The model under review builds one solid part; all positions refer to its coordinate system, in mm. A direction names the side the tool comes from. Round coordinates to 2 decimals unless told otherwise and drop trailing zeros. Loops run counter-clockwise (first coordinate to the right, second up) from the corner with the lowest first, then second, coordinate; pieces in that order, holes last. Notation, with made-up numbers: (58.25, 45) - (97.25, 45) arc R18 ccw to (97.25, 77) - close; hole circle Ø3 at (79, 20). An arc over 180 degrees is marked (long way). Answer as CSV lines item,"result".
Autodesk Inventor part; units mm, degrees
ref_plane "YZ Plane" through (0, 0, 0) normal (1, 0, 0) x (0, 1, 0)
ref_plane "XZ Plane" through (0, 0, 0) normal (0, 1, 0) x (-1, 0, 0)
ref_plane "XY Plane" through (0, 0, 0) normal (0, 0, 1) x (1, 0, 0)
sketch "Sketch1" plane through (0, 0, 0) normal (1, 0, 0) x (0, 1, 0)
  line L0 (15, 25) -> (-5, 25)
  line L1 (-5, 25) -> (-5, -25)
  line L2 (-5, -25) -> (15, -25)
  line L3 (15, -25) -> (0, -10)
  line L4 (0, -10) -> (0, 10)
  line L5 (0, 10) -> (15, 25)
  line L6 (0, 0) -> (-5, 0) construction
  circle A0 centre (5, -20) radius 2
  circle A1 centre (5, 20) radius 2
  dimension "d0" = 50
  dimension "d1" = 45
  dimension "d2" = 5
  dimension "d4" = 40
  dimension "d5" = 4
  dimension "d6" = 20
  dimension "d7" = 5
  dimension "d8" = 15
extrude "Extrusion1" add sketch "Sketch1" along normal blind 5
sketch "Sketch2" plane through (0, 0, 0) normal (-1, 0, 0) x (0, 0, 1)
  line L0 (25, -5) -> (-25, -5)
  line L1 (-25, -5) -> (25, -5)
  line L2 (25, -5) -> (25, 0)
  line L3 (25, 0) -> (-25, 0)
  line L4 (-25, 0) -> (-25, -5)
  point P0 (0, 0)
extrude "Extrusion2" add sketch "Sketch2" along normal blind 10
mirror "Mirror1" about plane through (-10, -2.5, 0) normal (-1, 0, 0)
sketch "Sketch3" plane through (0, 0, 10) normal (0, 1, 0) x (1, 0, 0)
  line L0 (-20, 0) -> (-20, -15) construction
  line L1 (0, 20) -> (5, 20) construction
  line L2 (-20, 0) -> (0, 20) construction
  line L3 (-20, 35) -> (-20, 20) construction
  line L4 (0, 0) -> (5, 0) construction
  line L5 (-20, 20) -> (0, 0) construction
  circle A0 centre (-10, 10) radius 2
  point P0 (0, 10)
  dimension "d13" = 4
extrude "Extrusion3" cut sketch "Sketch3" against normal blind 2
sketch "Sketch4" plane through (0, 0, 10) normal (0, 1, 0) x (1, 0, 0)
  circle A0 centre (-10, 10) radius 2
  circle A1 centre (-10, 10) radius 1
  point P0 (0, 10)
  dimension "d16" = 2
extrude "Extrusion4" cut sketch "Sketch4" against normal through all contours A1
equation "\"d7\" = 0.333333 * d8"
properties part number "lower fan mount"
1. Clearance check with flat-ended pins moving along their axes: pin 1 (1 mm diameter, centred on x = -3, z = 19.5, fed in from +Y); pin 2 (12 mm diameter, centred on y = 9, z = -17.5, fed in from -X); pin 3 (2 mm diameter, centred on x = -10, z = -0.5, fed in from +Y); pin 4 (3 mm diameter, centred on y = 2.5, z = 2.5, fed in from +X). State where each tip first meets the part, or that it passes through.
Numbers:
pin 1,"stops at y = 0"
pin 2,"stops at x = -25"
pin 3,"stops at y = -2"
pin 4,"passes through"
2. Take a section at A-A (y = 10.5). State the section outline as (x, z) points, plus the area to 3 significant figures.
Numbers:
outline,"(-25, -25) - (-20, -25) - (-20, -20.5) - (-25, -20.5) - close; (-25, 20.5) - (-20, 20.5) - (-20, 25) - (-25, 25) - close; (0, -25) - (5, -25) - (5, -20.5) - (0, -20.5) - close; (0, 20.5) - (5, 20.5) - (5, 25) - (0, 25) - close"
area,"90.0 mm²"
3. Draft analysis for pull direction X (two halves, no side actions). For faces 5 (the face through (5, -2, 0)), 6 (the face through (-20, 3, -21)), 7 (the face through (-7, -5, 0)), state which applies: +X half, -X half, draft (parallel to the pull), parting line (faces both ways), or undercut.
Numbers:
face 5,"+X half"
face 6,"undercut"
face 7,"draft"
4. Take a section at B-B (z = 20). State the section outline as (x, y) points.
Numbers:
outline,"(-25, -5) - (5, -5) - (5, 3) - (0, 3) - (0, 0) - (-20, 0) - (-20, 3) - (-25, 3) - close; (-25, 7) - (-20, 7) - (-20, 10) - (-25, 10) - close; (0, 7) - (5, 7) - (5, 10) - (0, 10) - close"
5. Take a section at C-C (x = -10). State the section outline as (y, z) points, plus the area to 3 significant figures.
Numbers:
outline,"(-5, -25) - (0, -25) - (0, -2) - (-2, -2) - (-2, -1) - (-5, -1) - close; (-5, 1) - (-2, 1) - (-2, 2) - (0, 2) - (0, 25) - (-5, 25) - close"
area,"236 mm²"
6. Take a section at D-D (y = 5). State how many separate pieces and enclosed holes the cut face has, plus the area to 3 significant figures.
Numbers:
separate pieces,"8"
enclosed holes,"0"
area,"120 mm²"
7. Tool access review of faces 1 (the face through (0, 4, -22)), 2 (the face through (-22, 7, -17)), 3 (the face through (-14, -2, -25)), 4 (the face through (-11.6, -1, 1.2)): name each direction out of +Z, -Z, +X, -X, +Y, -Y from which nothing blocks a thin tool from reaching the whole face with its end or side.
Numbers:
face 1,"+Z, -Z, +Y"
face 2,"+X, -X, +Y"
face 3,"-Z, +X, -X, +Y, -Y"
face 4,"+Y"
8. Wall thickness on probe 1 along Z at (x, y) = (-10, -0.9); probe 2 along Z at (x, y) = (2.3, 5); probe 3 along X at (y, z) = (5.75, -17): over which ranges is each line inside the solid? List them lowest first.
Numbers:
probe 1,"z = -25 to -2, 2 to 25"
probe 2,"z = -25 to -22, -18 to -15, 15 to 18, 22 to 25"
probe 3,"x = -25 to -20, 0 to 5"
